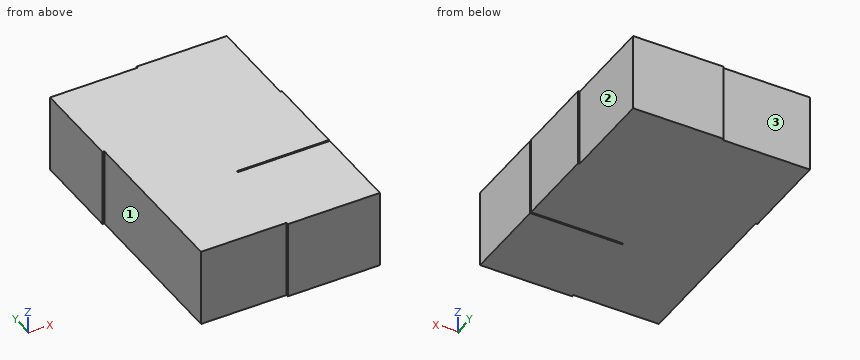
from build123d import *

# Parameters (mm, degrees)
F0_W     = 39.7309437394
F0_H     = 35.8594581485
F0_H_2   = 34.1520495713
F0_W_2   = 39.8523285985
F1_DEPTH = 25.4
F2_W     = 39.7309437394
F2_H     = 34.1520495713
F3_DEPTH = 25.4
F5_W     = 33.1652238965
F5_H     = 31.9460257888
F6_DEPTH = 30.226


with BuildPart() as f1:
    # F0 (on Top) → F1 (new body)
    with BuildSketch(Plane.XY):
        with Locations((-19.8654718697, 17.9297290742)):
            Rectangle(F0_W, F0_H)
        with Locations((-19.8654718697, -17.0760247856)):
            Rectangle(F0_W, F0_H_2)
        with Locations((19.9261642992, 17.9297290742)):
            Rectangle(F0_W_2, F0_H)
    extrude(amount=F1_DEPTH)

    # F2 (on face) → F3 (join)
    with BuildSketch(Plane.XY.offset(25.4)):
        with Locations((-19.8654718697, -17.0760247856)):
            Rectangle(F2_W, F2_H)
    extrude(amount=F3_DEPTH)


with BuildPart() as f6:
    # F5 (on Top) → F6 (new body)
    with BuildSketch(Plane.XY):
        with Locations((-16.5826119483, -15.9730128944)):
            Rectangle(F5_W, F5_H)
        Polygon((-33.1652238965, 0), (0, 0), (0, 35.6270745397), (-33.8673219085, 35.6270745397), (-33.8673219085, 0), align=None)
        Polygon((0, 35.6270745397), (0, 0), (35.113606602, 0), (35.113606602, 36.3328047097), (0, 36.3328047097), align=None)
        Polygon((35.113606602, 0), (0, 0), (0, -31.9460257888), (35.7213914394, -31.9460257888), (35.7213914394, 0), align=None)
        Polygon((0, -32.553806901), (0, -31.9460257888), (-33.1652238965, -31.9460257888), (-33.1652238965, -65.6626299024), (0, -65.6626299024), align=None)
        Polygon((35.7213914394, -32.553806901), (0, -32.553806901), (0, -65.6626299024), (0, -66.5416121483), (35.7213914394, -66.5416121483), align=None)
    extrude(amount=F6_DEPTH)


solid = f6.part
Verification items for the finished model (mm, model axes). Face numbers are marked on the shaded views. A direction names the side the tool comes from. Coordinates: 2 decimals unless noted, no trailing zeros. Order: outer loops, then holes, each group sorted by start corner. A loop starts at its lowest first (then second) coordinate and runs counter-clockwise, first axis right, second up. Notation, with made-up numbers: M 1,-1.5 L 37,-1.5 A15 cw 37,7.5 Z; hole C 62,-16.5 d3. An arc over 180 degrees is marked long. One line per item, written item: value. Start each with the question number.
Item 1: Sectioned sample at B-B (x = -21). Enter the section's corners in (y, z), then the cut area to 3 significant figures.
Item 2: Sectioned sample at A-A (z = 3). Enter the section's corners in (x, y).
Item 3: Access from +Z, -Z, +X, -X, +Y, -Y to the whole of each face (thin tool, end or side, straight path). Record for the marked faces 1, 2 and 3.
Item 4: Gauge pin test, flat ends, axial feed: pin 1 (8 mm diameter, centred on y = -11, z = 8, fed in from -X); pin 2 (15 mm diameter, centred on x = -22, z = 18, fed in from -Y); pin 3 (12 mm diameter, centred on y = 25.5, z = 18, fed in from +X). Record the tip position at first contact, or that the pin passes through.
Item 5: Scan lines: probe 1 along Y at (x, z) = (9.5, 10.5); probe 2 along Y at (x, z) = (-8, 21.5); probe 3 along X at (y, z) = (-38, 26). Record each from-to range of solid material in increasing order.
Conclusion:
1. outline: M -65.66,0 L 35.63,0 L 35.63,30.23 L -65.66,30.23 Z
1. area: 3,060 mm^2
2. outline: M -33.87,0 L -33.17,0 L -33.17,-65.66 L 0,-65.66 L 0,-66.54 L 35.72,-66.54 L 35.72,-32.55 L 0,-32.55 L 0,-31.95 L 35.72,-31.95 L 35.72,0 L 35.11,0 L 35.11,36.33 L 0,36.33 L 0,35.63 L -33.87,35.63 Z
3. face 1: +Z, -Z, -X, -Y
3. face 2: +Z, -Z, +X, +Y
3. face 3: +Z, -Z, -X, +Y
4. pin 1: stops at x = -33.17
4. pin 2: stops at y = -65.66
4. pin 3: stops at x = 35.11
5. probe 1: y = -66.54 to -32.55, -31.95 to 36.33
5. probe 2: y = -65.66 to 35.63
5. probe 3: x = -33.17 to 35.72
